The model under review builds one solid part; all positions refer to its coordinate system, in mm. A direction names the side the tool comes from. Round coordinates to 2 decimals unless told otherwise and drop trailing zeros. Loops run counter-clockwise (first coordinate to the right, second up) from the corner with the lowest first, then second, coordinate; pieces in that order, holes last. Notation, with made-up numbers: (52, 55.25) -> (88, 55.25) arc R28 ccw to (88, 82.25) -> close; hole circle Ø9 at (24, -38). An arc over 180 degrees is marked (long way). Use a Markdown table: item, result. Add a question column.
1) Wall thickness on probe 1 along X at (y, z) = (-686, 685); probe 2 along Z at (x, y) = (-685, -770); probe 3 along Y at (x, z) = (0, 185.5): over which ranges is each line inside the solid? List them lowest first.
2) Mouldability with a two-part tool opening along Y and no side actions: class faces 1 (the flat face through (-576, -533.4, 464)), 2 (the flat face through (68, 112, 171.45)), 3 (the flat face through (914.4, -684, 451)) as released by +Y, released by -Y, zero draft, split by the parting line, or undercut.
3) For faces 4 (the flat face through (182.88, -381, 424)), 5 (the flat face through (228.6, -322, 362)), 6 (the flat face through (-228.6, -322, 362)), list the 3-axis set-ups (+Z, -Z, +X, -X, +Y, -Y) from which the entire face can be reached by the end or side of a thin tool; tool diameter is ignored.
4) Consider section C-C on y = -729.5. Give the boundary of the cut face in (x, z), plus the area to 3 significant figures.
5) Insertion check: pin 1 (8 mm diameter, centred on y = -148.5, z = 152, fed in from +X); pin 2 (5 mm diameter, centred on x = 418, z = 299.5, fed in from +Y). Each pin has a flat end and moves straight along its axis. Give the tip position at first contact, or say it passes through.
6) Consider section D-D on y = 64.5. Give the boundary of the cut face in (x, z).
7) Consider section A-A on x = 685.8. Give the boundary of the cut face in (y, z), plus the area to 3 significant figures.
8) Consider section B-B on x = 0. Give the boundary of the cut face in (y, z), plus the area to 3 significant figures.
from build123d import *

# Parameters (mm, degrees)
EXTRUDE_1_DEPTH          = 228.6
CUT_EXTRUDE_1_DEPTH      = 624.723881217
CUT_EXTRUDE_1_DEPTH_BACK = 57.15
SKETCH_2_R               = 152.4
SKETCH_2_R_2             = 129.54
SKETCH_3_R               = 129.54
CUT_EXTRUDE_2_DEPTH      = 624.723881217
SKETCH_4_W               = 1828.8
SKETCH_4_H               = 914.4
EXTRUDE_2_DEPTH          = 304.8
RIB_START                = -45.72
RIB_11_DEPTH             = 45.72
SKETCH_6_R               = 114.3
CUT_EXTRUDE_3_DEPTH      = 1677.4


# Read off the part's stored shape, not the designer's step: 筋11
with BuildPart() as part:
    # 草图1 → 凸台-拉伸1 (new body)
    with BuildSketch(Plane.XY):
        with BuildLine():
            Line((-228.6, 0), (-228.6, -533.4))
            Line((-228.6, -533.4), (228.6, -533.4))
            Line((228.6, -533.4), (228.6, 0))
            ThreePointArc((228.6, 0), (0, 228.6), (-228.6, 0))
        make_face()
    extrude(amount=EXTRUDE_1_DEPTH)

    # 草图2 → 切除-拉伸1 (cut, two sides: drawn at the far end of the back side and taken through both)
    with BuildSketch(Plane.XY.offset(228.6).offset(-CUT_EXTRUDE_1_DEPTH_BACK)):
        with Locations(Location((0, 0, 0), (0, 0, 180))):
            Circle(SKETCH_2_R)
        with Locations(Location((0, 0, 0), (0, 0, 180))):
            Circle(SKETCH_2_R_2, mode=Mode.SUBTRACT)
    extrude(amount=CUT_EXTRUDE_1_DEPTH + CUT_EXTRUDE_1_DEPTH_BACK, mode=Mode.SUBTRACT)

    # 草图3 → 切除-拉伸2 (cut, through all)
    with BuildSketch(Plane.XY.offset(228.6)):
        Circle(SKETCH_3_R)
    extrude(amount=-CUT_EXTRUDE_2_DEPTH, mode=Mode.SUBTRACT)

    # 草图4 → 凸台-拉伸2 (add)
    with BuildSketch(Plane.XZ.offset(533.4)):
        with Locations((0, 457.2)):
            Rectangle(SKETCH_4_W, SKETCH_4_H)
    extrude(amount=EXTRUDE_2_DEPTH)

    # 筋11 outline → 筋11 (add)
    with BuildSketch(Plane(origin=(228.6, 0, 0), x_dir=(0, 0, -1), z_dir=(1, 0, 0)).offset(RIB_START)):
        Polygon((-228.6, -533.4), (-228.6, 0), (-914.4, -533.4), align=None)
    rib_11 = extrude(amount=RIB_11_DEPTH)

    # 镜向1: 筋11 across plane
    add(rib_11.mirror(Plane(origin=(0, 0, 0), x_dir=(0, 0, 1), z_dir=(1, 0, 0))))

    # 草图6 → 切除-拉伸3 (cut, through all)
    with BuildSketch(Plane.XZ.offset(838.2)):
        with Locations(Location((-685.8, 685.8, 0), (0, 0, 270))):
            Circle(SKETCH_6_R)
        with Locations(Location((-685.8, 228.6, 0), (0, 0, 90))):
            Circle(SKETCH_6_R)
        with Locations(Location((685.8, 228.6, 0), (0, 0, 270))):
            Circle(SKETCH_6_R)
        with Locations(Location((685.8, 685.8, 0), (0, 0, 90))):
            Circle(SKETCH_6_R)
    extrude(amount=-CUT_EXTRUDE_3_DEPTH, mode=Mode.SUBTRACT)


solid = part.part
Result set:
| question | item | result |
|---|---|---|
| 1 | probe 1 | -914.4 to -800.1, -571.5 to 571.5, 800.1 to 914.4 |
| 1 | probe 2 | 0 to 114.3, 342.9 to 571.5, 800.1 to 914.4 |
| 1 | probe 3 | -838.2 to -152.4, 152.4 to 228.6 |
| 2 | face 1 | released by +Y |
| 2 | face 2 | undercut |
| 2 | face 3 | zero draft |
| 3 | face 4 | +Z, +Y |
| 3 | face 5 | +Z, -Z, +X, +Y |
| 3 | face 6 | +Z, -Z, -X, +Y |
| 4 | outline | (-914.4, 0) -> (914.4, 0) -> (914.4, 914.4) -> (-914.4, 914.4) -> close; hole circle Ø228.6 at (-685.8, 228.6); hole circle Ø228.6 at (-685.8, 685.8); hole circle Ø228.6 at (685.8, 228.6); hole circle Ø228.6 at (685.8, 685.8) |
| 4 | area | 1,510,000 mm2 |
| 5 | pin 1 | x = 228.6 |
| 5 | pin 2 | y = -533.4 |
| 6 | outline | (-219.31, 0) -> (-112.34, 0) -> (-112.34, 171.45) -> (-138.08, 171.45) -> (-138.08, 228.6) -> (-219.31, 228.6) -> close; (112.34, 0) -> (219.31, 0) -> (219.31, 228.6) -> (138.08, 228.6) -> (138.08, 171.45) -> (112.34, 171.45) -> close |
| 7 | outline | (-838.2, 0) -> (-533.4, 0) -> (-533.4, 114.3) -> (-838.2, 114.3) -> close; (-838.2, 342.9) -> (-533.4, 342.9) -> (-533.4, 571.5) -> (-838.2, 571.5) -> close; (-838.2, 800.1) -> (-533.4, 800.1) -> (-533.4, 914.4) -> (-838.2, 914.4) -> close |
| 7 | area | 139,000 mm2 |
| 8 | outline | (-838.2, 0) -> (-129.54, 0) -> (-129.54, 171.45) -> (-152.4, 171.45) -> (-152.4, 228.6) -> (-533.4, 228.6) -> (-533.4, 914.4) -> (-838.2, 914.4) -> close; (129.54, 0) -> (228.6, 0) -> (228.6, 228.6) -> (152.4, 228.6) -> (152.4, 171.45) -> (129.54, 171.45) -> close |
| 8 | area | 391,000 mm2 |
